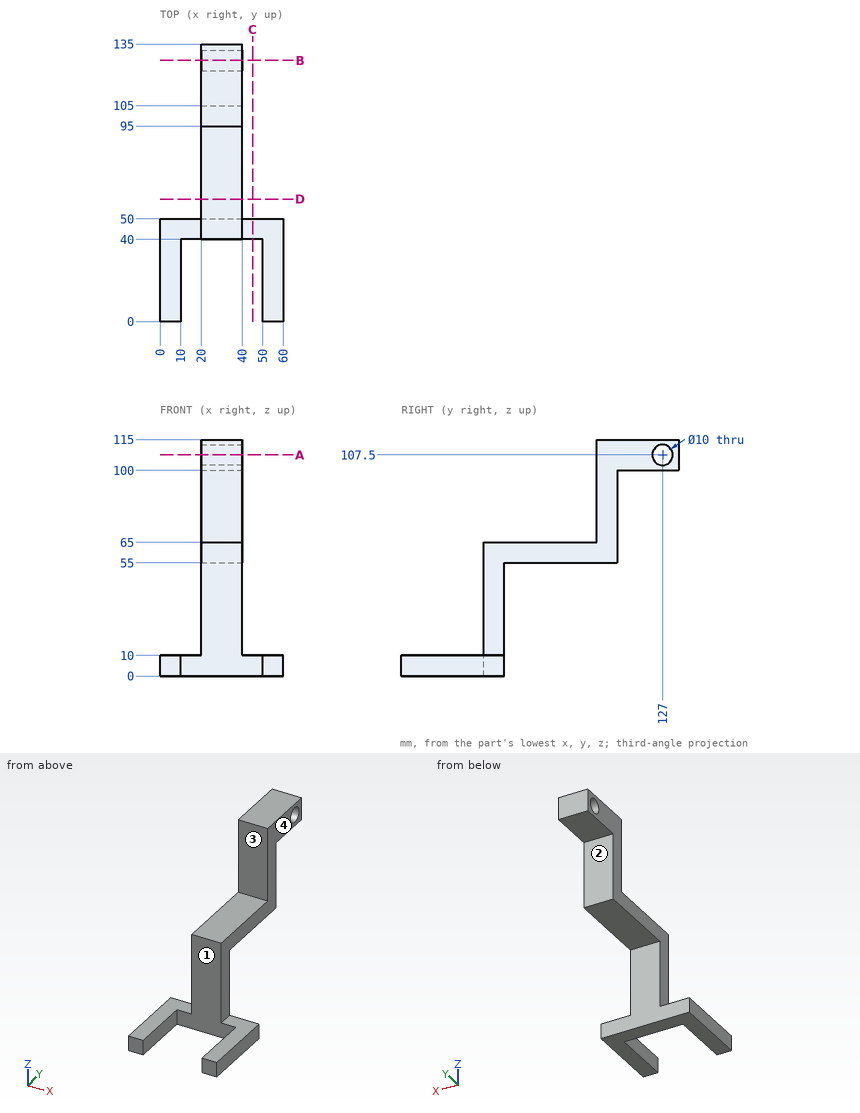
Study the drawing (mm; zero at the part's minimum x, y, z) and answer. A direction names the side the tool comes from. Round coordinates to 2 decimals unless told otherwise and drop trailing zeros. Loops run counter-clockwise (first coordinate to the right, second up) from the corner with the lowest first, then second, coordinate; pieces in that order, holes last.
Q1. Section B-B, the plane y = 127 is taken. Determine the outline of the cut face in (x, z), then the cut area to 3 significant figures.
Q2. Section A-A, the plane z = 107.5 is taken. Determine the outline of the cut face in (x, y).
Q3. Which of the six approach directions +Z, -Z, +X, -X, +Y, -Y give full straight-line access (tool end or side, diameter ignored) to the marked faces 1, 2, 3 and 4?
Q4. Section D-D, the plane y = 59.5 is taken. Determine the outline of the cut face in (x, z), then the cut area to 3 significant figures.
Q5. Section C-C, the plane x = 45 is taken. Determine the outline of the cut face in (y, z), then the cut area to 3 significant figures.
Q6. Find the intervals of material crossed by line 1 (Y direction, x = 27, z = 107.5); line 2 (Y direction, x = 13.5, z = 7); line 3 (X direction, y = 105.5, z = 103.5), in increasing order.
Q7. Given pin 1 Ø12 at (y, z) = (41, 69) entering from -X; pin 2 Ø10 at (x, y) = (26, 122.5) entering from -Z; pin 3 Ø6 at (x, y) = (25.5, 59.5) entering from +Z, each flat-ended and moving along its own axis, determine where each tip first touches the part or whether it passes through.
Completed:
1. outline: (20, 100) - (40, 100) - (40, 102.5) - (20, 102.5) - close; (20, 112.5) - (40, 112.5) - (40, 115) - (20, 115) - close
1. area: 100 mm2
2. outline: (20, 95) - (40, 95) - (40, 122) - (20, 122) - close; (20, 132) - (40, 132) - (40, 135) - (20, 135) - close
3. face 1: +Z, -Z, -Y
3. face 2: -Z, +X, -X, +Y
3. face 3: +Z, +X, -X, -Y
3. face 4: +Z, +X, +Y, -Y
4. outline: (20, 55) - (40, 55) - (40, 65) - (20, 65) - close
4. area: 200 mm2
5. outline: (40, 0) - (50, 0) - (50, 10) - (40, 10) - close
5. area: 100 mm2
6. line 1: y = 95 to 122, 132 to 135
6. line 2: y = 40 to 50
6. line 3: x = 20 to 40
7. pin 1: stops at x = 20
7. pin 2: stops at z = 100
7. pin 3: stops at z = 65
